from build123d import *

# Parameters (mm, degrees)
SKETCH_1_W          = 20
SKETCH_1_H          = 20
SKETCH_1_W_2        = 18
SKETCH_1_H_2        = 18
EXTRUDE_1_DEPTH     = 136
SKETCH_2_R          = 3
CUT_EXTRUDE_1_DEPTH = 200
SKETCH_3_R          = 2
SKETCH_3_R_2        = 1.65
CUT_EXTRUDE_2_DEPTH = 138.825977232


with BuildPart() as part:
    # 草图1 → 凸台-拉伸1 (new, symmetric)
    with BuildSketch(Plane(origin=(0, 0, 0), x_dir=(1, 0, 0), z_dir=(0, 1, 0))):
        Rectangle(SKETCH_1_W, SKETCH_1_H)
        Rectangle(SKETCH_1_W_2, SKETCH_1_H_2, mode=Mode.SUBTRACT)
    extrude(amount=EXTRUDE_1_DEPTH, both=True)

    # 草图2 → 切除-拉伸1 (cut)
    with BuildSketch(Plane.XY.offset(10)):
        with Locations((-2.5, 105)):
            Circle(SKETCH_2_R)
        with Locations((2.5, 117)):
            Circle(SKETCH_2_R)
    extrude(amount=-CUT_EXTRUDE_1_DEPTH, mode=Mode.SUBTRACT)

    # 草图3 → 切除-拉伸2 (cut, through all)
    with BuildSketch(Plane.ZY.offset(10)):
        with Locations((0, -128)):
            Circle(SKETCH_3_R)
        with Locations((0, 57.2863231)):
            Circle(SKETCH_3_R_2)
        with Locations((0, 67.2863231)):
            Circle(SKETCH_3_R_2)
        with Locations((0, -12.7136769)):
            Circle(SKETCH_3_R_2)
        with Locations((0, -22.7136769)):
            Circle(SKETCH_3_R_2)
        with Locations((0, 37.2863231)):
            Circle(SKETCH_3_R_2)
        with Locations((0, 7.2863231)):
            Circle(SKETCH_3_R_2)
    extrude(amount=-CUT_EXTRUDE_2_DEPTH, mode=Mode.SUBTRACT)


solid = part.part
Build history of the part. All positions in model axes, mm. A direction names the side the tool comes from. Round coordinates to 2 decimals unless told otherwise and drop trailing zeros. Loops run counter-clockwise (first coordinate to the right, second up) from the corner with the lowest first, then second, coordinate; pieces in that order, holes last. Notation, with made-up numbers: (71, 66.25) -> (107, 66.25) arc R18 cw to (107, 91.25) -> close; hole circle Ø9 at (-20, 30). An arc over 180 degrees is marked (long way). One line per item, written item: value. Start each with the question number.
Q1. Two-plate mould, pull along X, no slides. Class faces 3 (the face through (-10, 2, 0)), 4 (the face through (-0.8, -136, 9.6)), 5 (the face through (10, 2, 0)), 6 (the face through (-3.15, 102.07, -9.49)): released by +X, released by -X, zero draft, split by the parting line, or undercut.
Q2. 3-axis set-ups, long thin cutter, end or side, ignore diameter. For faces 1 (the face through (0, 2, 10)), 2 (the face through (9, 2, 0)): which of +Z, -Z, +X, -X, +Y, -Y reach the whole face in a straight line?
Q3. Drop a flat-ended pin along its axis: pin 1 Ø3 at (y, z) = (37.29, 0) entering from -X. Give the stop position or say it passes through.
Q4. Probe line 1 along X through (y, z) = (-31, 3.5); line 2 along Y through (x, z) = (2.5, -9.4). List the from-to ranges inside material, lowest first.
Q5. Cut at A-A on y = -107. List the corners of the cut face in (x, z), plus the area to 3 significant figures.
Q6. Cut at B-B on x = -3. List the corners of the cut face in (y, z).
Computed:
1. face 3: released by -X
1. face 4: zero draft
1. face 5: released by +X
1. face 6: undercut
2. face 1: +Z, +X, -X, +Y, -Y
2. face 2: +Y, -Y
3. pin 1: through
4. line 1: -10 to -9, 9 to 10
4. line 2: -136 to 114, 120 to 136
5. outline: (-10, -10) -> (10, -10) -> (10, 10) -> (-10, 10) -> close; hole (-9, -9) -> (9, -9) -> (9, 9) -> (-9, 9) -> close
5. area: 76.0 mm²
6. outline: (-136, -10) -> (102.04, -10) -> (102.04, -9) -> (-136, -9) -> close; (-136, 9) -> (102.04, 9) -> (102.04, 10) -> (-136, 10) -> close; (107.96, -10) -> (136, -10) -> (136, -9) -> (107.96, -9) -> close; (107.96, 9) -> (136, 9) -> (136, 10) -> (107.96, 10) -> close
